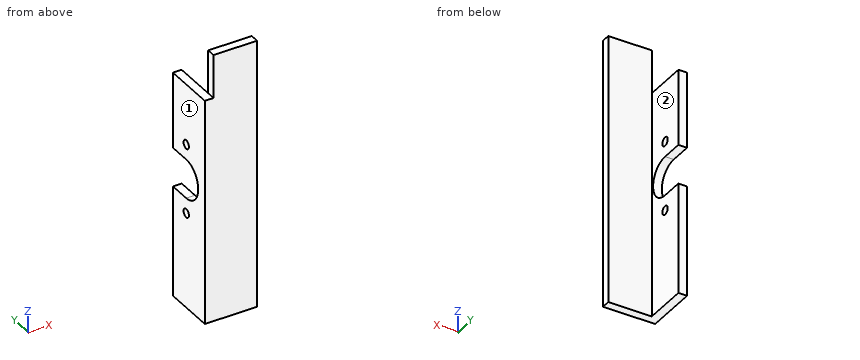
from build123d import *

# Parameters (mm, degrees)
BOSS_EXTRUDE1_DEPTH = 196.85
SKETCH2_W           = 31.75
SKETCH2_H           = 38.1
CUT_EXTRUDE1_DEPTH  = 6.35
SKETCH3_R           = 3.175
CUT_EXTRUDE2_DEPTH  = 7.35


with BuildPart() as part:
    # Sketch1 → Boss-Extrude1 (new body)
    with BuildSketch(Plane.XY):
        Polygon((0, 0), (0, 38.1), (6.35, 38.1), (6.35, 6.35), (38.1, 6.35), (38.1, 0), align=None)
    extrude(amount=BOSS_EXTRUDE1_DEPTH)

    # Sketch2 → Cut-Extrude1 (cut)
    with BuildSketch(Plane(origin=(0, 0, 0), x_dir=(0, 0, -1), z_dir=(1, 0, 0))):
        with Locations((-180.975, 19.05)):
            Rectangle(SKETCH2_W, SKETCH2_H)
    extrude(amount=CUT_EXTRUDE1_DEPTH, mode=Mode.SUBTRACT)

    # Sketch3 → Cut-Extrude2 (cut, through all)
    with BuildSketch(Plane(origin=(6.35, 0, 0), x_dir=(0, 0, -1), z_dir=(1, 0, 0))):
        with Locations((-120.65, 22.225)):
            Circle(SKETCH3_R)
        with Locations((-69.85, 22.225)):
            Circle(SKETCH3_R)
        with BuildLine():
            Line((-109.5375, 22.225), (-109.5375, 38.1))
            Line((-109.5375, 38.1), (-80.9625, 38.1))
            Line((-80.9625, 38.1), (-80.9625, 22.225))
            ThreePointArc((-80.9625, 22.225), (-95.25, 7.9375), (-109.5375, 22.225))
        make_face()
    extrude(amount=-CUT_EXTRUDE2_DEPTH, mode=Mode.SUBTRACT)


solid = part.part
Here's how the part is built. I have some questions about the finished solid (model axes, mm). Face numbers are marked on the shaded views. A direction names the side the tool comes from. Round coordinates to 2 decimals unless told otherwise and drop trailing zeros. Order: outer loops, then holes, each group sorted by start corner. A loop starts at its lowest first (then second) coordinate and runs counter-clockwise, first axis right, second up. Notation, with made-up numbers: (31, -17.75) -> (78, -17.75) arc R18 cw to (78, 10.25) -> close; hole circle Ø10 at (-21, 55). An arc over 180 degrees is marked (long way). Return JSON: item names as keys, results as strings.
Q1. Which directions (+Z, -Z, +X, -X, +Y, -Y) give clear straight access to the entire face, cutting with the end or side of a thin tool? Please do the marked faces 1 and 2.
Filled sheet:
{"face 1": "+Z, -Z, -X, +Y, -Y", "face 2": "+Z, -Z, +X, +Y"}
Q2. If we section it at C-C on y = 34: List the corners of the cut face in (x, z) for me.
Filled sheet:
{"outline": "(0, 0) -> (6.35, 0) -> (6.35, 80.96) -> (0, 80.96) -> close; (0, 109.54) -> (6.35, 109.54) -> (6.35, 165.1) -> (0, 165.1) -> close"}
Q3. If we section it at B-B on z = 120.65: List the corners of the cut face in (x, y) for me, plus the area to 3 significant figures.
Filled sheet:
{"outline": "(0, 0) -> (38.1, 0) -> (38.1, 6.35) -> (6.35, 6.35) -> (6.35, 19.05) -> (0, 19.05) -> close; (0, 25.4) -> (6.35, 25.4) -> (6.35, 38.1) -> (0, 38.1) -> close", "area": "403 mm^2"}
Q4. I need wall thicknesses on line 1 along Z through (x, y) = (4.5, 30); line 2 along X through (y, z) = (12, 83). Which ranges of each line are inside material? Lowest first, please. Write a range as from..to.
Filled sheet:
{"line 1": "z = 0..80.96, 109.54..165.1", "line 2": "x = 0..6.35"}
Q5. If we section it at A-A on x = 2: Give the number of separate pieces and of enclosed holes in the cut face, plus the area to 3 significant figures.
Filled sheet:
{"separate pieces": "1", "enclosed holes": "2", "area": "5,450 mm^2"}
Q6. If we section it at D-D on z = 68.5: List the corners of the cut face in (x, y) for me, plus the area to 3 significant figures.
Filled sheet:
{"outline": "(0, 0) -> (38.1, 0) -> (38.1, 6.35) -> (6.35, 6.35) -> (6.35, 19.35) -> (0, 19.35) -> close; (0, 25.1) -> (6.35, 25.1) -> (6.35, 38.1) -> (0, 38.1) -> close", "area": "407 mm^2"}
Q7. For pin 1 Ø5 at (x, y) = (4.5, 34) entering from +Z; pin 2 Ø10 at (x, y) = (13.5, 21) entering from +Z; pin 3 Ø12 at (x, z) = (27, 164) entering from +Y; pin 4 Ø1.9 at (y, z) = (2, 183.5) entering from -X, each with a flat end and sliding along its axis, tell me the tip position at first contact or that it passes through.
Filled sheet:
{"pin 1": "stops at z = 165.1", "pin 2": "passes through", "pin 3": "stops at y = 6.35", "pin 4": "stops at x = 6.35"}
